Input: part model. Units: mm. Frame: model coordinates. Coordinates: 2 decimals unless noted, no trailing zeros. Loops run counter-clockwise (first coordinate to the right, second up) from the corner with the lowest first, then second, coordinate; pieces in that order, holes last.
```python
from build123d import *

# Parameters (mm, degrees)
SKETCH1_W           = 42
SKETCH1_H           = 42
BOSS_EXTRUDE1_DEPTH = 4


with BuildPart() as part:
    # Sketch1 → Boss-Extrude1 (new body)
    with BuildSketch(Plane(origin=(0, 0, 0), x_dir=(1, 0, 0), z_dir=(0, 1, 0))):
        Polygon((-82.9, -82.9), (-82.9, -103), (82.9, -103), (82.9, -82.9), (103, -82.9), (103, 82.9), (82.9, 82.9), (82.9, 103), (-82.9, 103), (-82.9, 82.9), (-103, 82.9), (-103, -82.9), align=None)
        Rectangle(SKETCH1_W, SKETCH1_H, mode=Mode.SUBTRACT)
        Rectangle(SKETCH1_W, SKETCH1_H)
    extrude(amount=BOSS_EXTRUDE1_DEPTH)


solid = part.part
```
Item 1: Contact query for flat-ended pins moving along their axis: P1, Ø2, axis at y = 1, z = 90, coming from the -X side; P2, Ø2, axis at x = 89.5, y = 2, coming from the +Z side; P3, Ø8, axis at x = 53, z = -5, coming from the -Y side; P4, Ø1.2, axis at y = 2.5, z = 94, coming from the +X side. Output: stop coordinate, or through.
Result:
P1: stops at x = -82.9
P2: stops at z = 82.9
P3: stops at y = 0
P4: stops at x = 82.9
Item 2: Section query B-B (z = 87.5). Output: boundary loops of the cut face in (x, y), then the cut area to 3 significant figures.
Result:
outline: (-82.9, 0) - (82.9, 0) - (82.9, 4) - (-82.9, 4) - close
area: 663 mm2
Item 3: Section query A-A (y = 2.55). Output: boundary loops of the cut face in (x, z).
Result:
outline: (-103, -82.9) - (-82.9, -82.9) - (-82.9, -103) - (82.9, -103) - (82.9, -82.9) - (103, -82.9) - (103, 82.9) - (82.9, 82.9) - (82.9, 103) - (-82.9, 103) - (-82.9, 82.9) - (-103, 82.9) - close
Item 4: Line query: L1, parallel to Z at x = 86.5, y = 1.15. Output: solid intervals per line, ascending.
Result:
L1: z = -82.9 to 82.9
